Here's the drawing with two shaded views (mm, measured from the low corner). I have some questions. A direction names the side the tool comes from. Give positions to 0.01 mm unless a question says otherwise; leave off trailing zeros. Order: outer loops, then holes, each group sorted by start corner. A loop starts at its lowest first (then second) coordinate and runs counter-clockwise, first axis right, second up. Notation, with made-up numbers: (5, 42) - (60, 42) arc R5 cw to (60, 50) - close; hole circle Ø7 at (50.25, 36). An arc over 180 degrees is marked (long way). Use one line per item in the form item = value. Start each with the question number.
1) Suppose I cut it at A-A, the plane z = 3.3. Write out the boundary of the cut face in (x, y) (3 decimals), and give its area (3 significant figures).
2) Suppose I cut it at B-B, the plane x = 3.5. Write out the boundary of the cut face in (y, z).
3) Which directions (+Z, -Z, +X, -X, +Y, -Y) give clear straight access to the entire face, cutting with the end or side of a thin tool? Please do the marked faces 1, 2 and 3.
4) Suppose I cut it at D-D, the plane x = 19.5. Write out the boundary of the cut face in (y, z) (3 decimals), and give its area (3 significant figures).
5) Suppose I cut it at C-C, the plane y = 6.5. Write out the boundary of the cut face in (x, z), and give its area (3 significant figures).
6) Please list where these lines run through material, in increasing order: probe 1 along Y at (x, z) = (19.25, 0.2) (3 decimals); probe 2 along X at (y, z) = (57.5, 2.95); probe 3 along X at (y, z) = (78.5, 4.4).
7) For pin 1 (1.5 mm diameter, centred on x = 10, z = 3.5, fed in from -Y); pin 2 (2.5 mm diameter, centred on y = 72.5, z = 3, fed in from +X); pin 3 (1.5 mm diameter, centred on x = 19.5, z = 0.5, fed in from +Y) (3 decimals), each with a flat end and sliding along its axis, tell me the tip position at first contact or that it passes through.
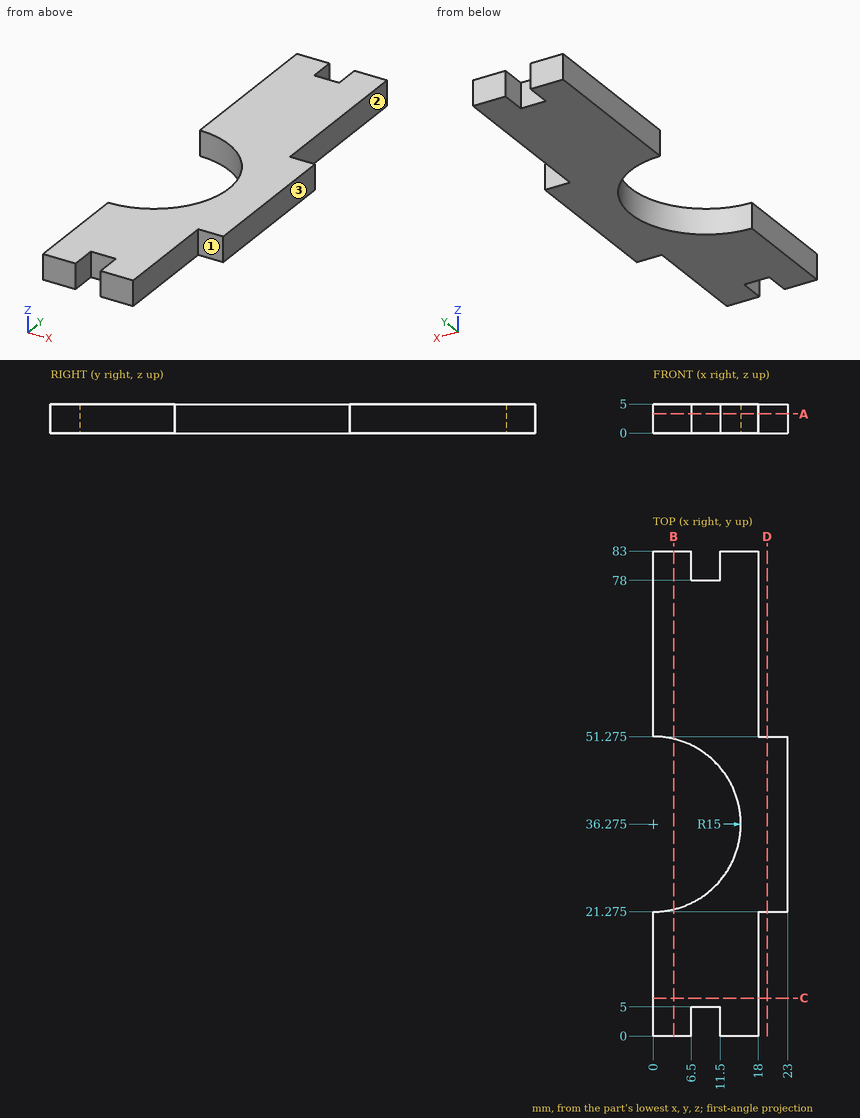
Result sheet:
q1.outline = (0, 0) - (6.5, 0) - (6.5, 5) - (11.5, 5) - (11.5, 0) - (18, 0) - (18, 21.275) - (23, 21.275) - (23, 51.275) - (18, 51.275) - (18, 83) - (11.5, 83) - (11.5, 78) - (6.5, 78) - (6.5, 83) - (0, 83) - (0, 51.275) arc R15 cw to (0, 21.275) - close
q1.area = 1,240 mm²
q2.outline = (0, 0) - (21.69, 0) - (21.69, 5) - (0, 5) - close; (50.86, 0) - (83, 0) - (83, 5) - (50.86, 5) - close
q3.face_1 = +Z, -Z, +X, -Y
q3.face_2 = +Z, -Z, +X, +Y
q3.face_3 = +Z, -Z, +X, +Y, -Y
q4.outline = (21.275, 0) - (51.275, 0) - (51.275, 5) - (21.275, 5) - close
q4.area = 150 mm²
q5.outline = (0, 0) - (18, 0) - (18, 5) - (0, 5) - close
q5.area = 90.0 mm²
q6.probe_1 = 21.275 to 51.275
q6.probe_2 = 0 to 18
q6.probe_3 = 0 to 6.5, 11.5 to 18
q7.pin_1 = 5
q7.pin_2 = 18
q7.pin_3 = 51.275
